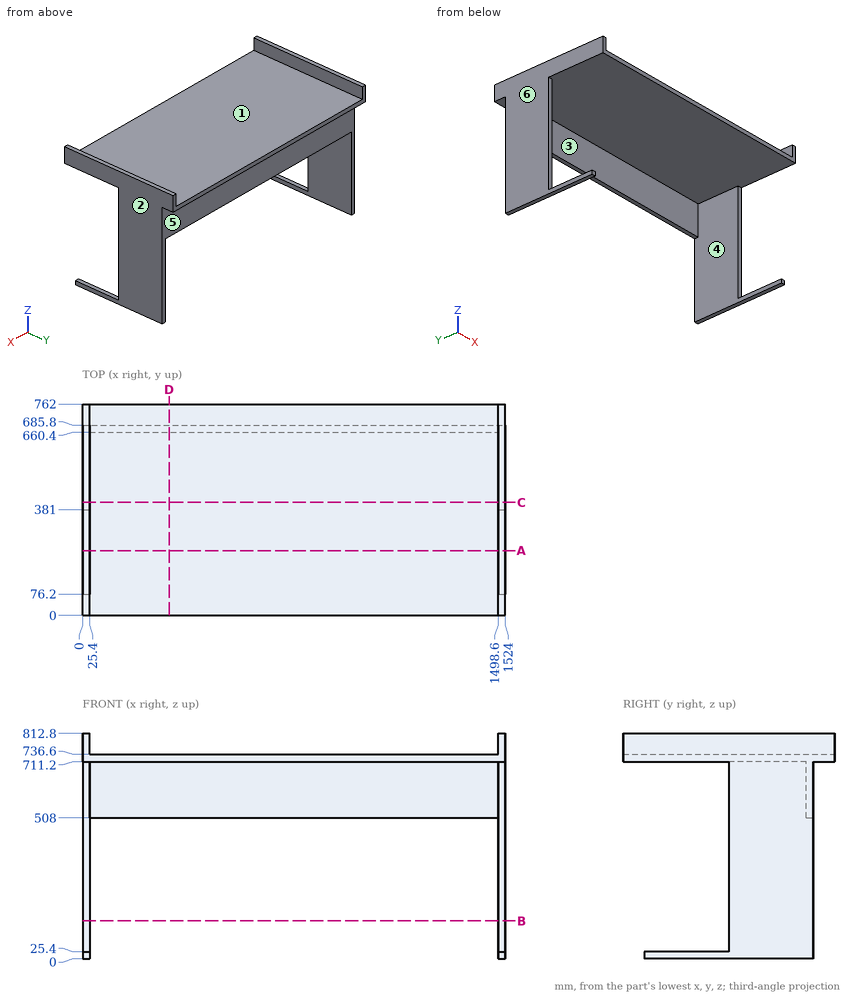
Here's the drawing with two shaded views (mm, measured from the low corner). I have some questions. A direction names the side the tool comes from. Coordinates: 2 decimals unless noted, no trailing zeros. Loops run counter-clockwise (first coordinate to the right, second up) from the corner with the lowest first, then second, coordinate; pieces in that order, holes last. Notation, with made-up numbers: M -12.75,-27.5 L 42.25,-27.5 A14 ccw 42.25,-0.5 Z; hole C 27.5,65 d1. An arc over 180 degrees is marked long. Put each result on its own line as item: value. Start each with the question number.
(1) We'd pull the mould along X, two halves only. Please class the marked faces 4, 5 and 6: +X half, -X half, draft (parallel to the pull), parting line (faces both ways), or undercut.
(2) I need wall thicknesses on probe 1 along X at (y, z) = (621, 366.5); probe 2 along Z at (x, y) = (192, 242.5); probe 3 along Y at (x, z) = (986, 669.5). Which ranges of each line are inside material? Lowest first, please.
(3) Imagine slicing it at D-D on x = 312. List the corners of the cut face in (y, z) for me.
(4) Imagine slicing it at C-C on y = 407. List the corners of the cut face in (x, z) for me, and give its area (3 significant figures).
(5) Imagine slicing it at B-B on z = 137. List the corners of the cut face in (x, y) for me, and give its area (3 significant figures).
(6) Which directions (+Z, -Z, +X, -X, +Y, -Y) give clear straight access to the entire face, cutting with the end or side of a thin tool? Please do the marked faces 1, 2 and 3.
(7) Imagine slicing it at A-A on y = 233. List the corners of the cut face in (x, z) for me.
(8) Will these pins go through, and if not, where does the flat tip stop? pin 1 Ø7.5 at (x, z) = (13.5, 407) entering from -Y; pin 2 Ø6 at (x, y) = (839, 184) entering from -Z; pin 3 Ø7.5 at (x, y) = (687.5, 673.5) entering from -Z.
Worked answers:
1. face 4: undercut
1. face 5: draft
1. face 6: -X half
2. probe 1: x = 0 to 25.4, 1498.6 to 1524
2. probe 2: z = 711.2 to 736.6
2. probe 3: y = 660.4 to 685.8
3. outline: M 0,711.2 L 660.4,711.2 L 660.4,508 L 685.8,508 L 685.8,711.2 L 762,711.2 L 762,736.6 L 0,736.6 Z
4. outline: M 0,0 L 25.4,0 L 25.4,711.2 L 1498.6,711.2 L 1498.6,0 L 1524,0 L 1524,812.8 L 1498.6,812.8 L 1498.6,736.6 L 25.4,736.6 L 25.4,812.8 L 0,812.8 Z
4. area: 78,700 mm2
5. outline: M 0,381 L 25.4,381 L 25.4,685.8 L 0,685.8 Z; M 1498.6,381 L 1524,381 L 1524,685.8 L 1498.6,685.8 Z
5. area: 15,500 mm2
6. face 1: +Z, +Y, -Y
6. face 2: +Z, -Z, +X, +Y, -Y
6. face 3: -Z, -Y
7. outline: M 0,0 L 25.4,0 L 25.4,25.4 L 0,25.4 Z; M 0,711.2 L 1524,711.2 L 1524,812.8 L 1498.6,812.8 L 1498.6,736.6 L 25.4,736.6 L 25.4,812.8 L 0,812.8 Z; M 1498.6,0 L 1524,0 L 1524,25.4 L 1498.6,25.4 Z
8. pin 1: stops at y = 381
8. pin 2: stops at z = 711.2
8. pin 3: stops at z = 508
